```python
from build123d import *

# Parameters (mm, degrees)
SKETCH1_W           = 50.8
SKETCH1_H           = 25.4
BOSS_EXTRUDE2_DEPTH = 25.4
SKETCH3_R           = 5.08
BOSS_EXTRUDE3_DEPTH = 12.7
BOSS_EXTRUDE4_START = 50.8
BOSS_EXTRUDE4_DEPTH = 12.7
CUT_EXTRUDE1_START  = 58.42
CUT_EXTRUDE1_DEPTH  = 2.54
FILLET8_R           = 2.54


with BuildPart() as part:
    # Sketch1 → Boss-Extrude2 (new body)
    with BuildSketch(Plane(origin=(0, 0, 0), x_dir=(1, 0, 0), z_dir=(0, 1, 0))):
        with Locations((25.4, 12.7)):
            Rectangle(SKETCH1_W, SKETCH1_H)
    extrude(amount=BOSS_EXTRUDE2_DEPTH)

    # Sketch3 → Boss-Extrude3 (add)
    with BuildSketch(Plane.XY):
        with Locations(Location((12.7, 12.7, 0), (0, 0, 180))):
            Circle(SKETCH3_R)
        with Locations(Location((38.1, 12.7, 0), (0, 0, 180))):
            Circle(SKETCH3_R)
    extrude(amount=BOSS_EXTRUDE3_DEPTH)

    # Sketch4 → Boss-Extrude4 (add)
    with BuildSketch(Plane(origin=(0, 0, 0), x_dir=(0, 0, -1), z_dir=(1, 0, 0)).offset(BOSS_EXTRUDE4_START)):
        with BuildLine():
            Line((-6.35, 12.7), (6.35, 12.7))
            ThreePointArc((6.35, 12.7), (0, 6.35), (-6.35, 12.7))
        make_face()
    extrude(amount=BOSS_EXTRUDE4_DEPTH)

    # Sketch24 → Cut-Extrude1 (cut)
    with BuildSketch(Plane(origin=(0, 0, 0), x_dir=(0, 0, -1), z_dir=(1, 0, 0)).offset(CUT_EXTRUDE1_START)):
        with BuildLine():
            Line((-6.35, 12.7), (6.35, 12.7))
            ThreePointArc((6.35, 12.7), (0, 6.35), (-6.35, 12.7))
        make_face()
        with BuildLine():
            Line((-4.824854626, 11.43), (5.012523073, 11.43))
            ThreePointArc((5.012523073, 11.43), (0.093834223, 7.62), (-4.824854626, 11.43))
        make_face(mode=Mode.SUBTRACT)
    extrude(amount=CUT_EXTRUDE1_DEPTH, mode=Mode.SUBTRACT)

    # Fillet8
    fillet8_edges = [part.edges().sort_by_distance(p)[0] for p in [
        (50.8, 8.209871939, -4.490128061),
    ]]
    fillet(fillet8_edges, radius=FILLET8_R)


solid = part.part
```
CAD build for the part. Positions are in the model's coordinates, mm. A direction names the side the tool comes from. Round coordinates to 2 decimals unless told otherwise and drop trailing zeros. Order: outer loops, then holes, each group sorted by start corner. A loop starts at its lowest first (then second) coordinate and runs counter-clockwise, first axis right, second up. Notation, with made-up numbers: (34.25, 48.25) -> (68.25, 48.25) arc R12 ccw to (68.25, 60.25) -> close; hole circle Ø6 at (9, 3.5). An arc over 180 degrees is marked (long way). One line per question, with ' | ' between items.
Q1. Slice it at B-B (z = -20.5). Write the cut outline in (x, y).
Completed:
outline: (0, 0) -> (50.8, 0) -> (50.8, 25.4) -> (0, 25.4) -> close
Q2. Slice it at D-D (x = 13.5). Write the cut outline in (y, z), then the cut area to 3 significant figures.
Completed:
outline: (0, -25.4) -> (25.4, -25.4) -> (25.4, 0) -> (17.72, 0) -> (17.72, 12.7) -> (7.68, 12.7) -> (7.68, 0) -> (0, 0) -> close | area: 773 mm^2
Q3. Slice it at A-A (x = 38.1). Write the cut outline in (y, z), then the cut area to 3 significant figures.
Completed:
outline: (0, -25.4) -> (25.4, -25.4) -> (25.4, 0) -> (17.78, 0) -> (17.78, 12.7) -> (7.62, 12.7) -> (7.62, 0) -> (0, 0) -> close | area: 774 mm^2
Q4. Drop flat-ended pins along their axis: pin 1 (4 mm diameter, centred on x = 55, z = -1.5, fed in from +Y); pin 2 (3 mm diameter, centred on y = 10.5, z = 2, fed in from -X); pin 3 (5 mm diameter, centred on x = 32.5, z = 8, fed in from +Y). Give the stop position or say it passes through.
Completed:
pin 1: stops at y = 12.7 | pin 2: stops at x = 7.67 | pin 3: stops at y = 16.72
Q5. Probe probe 1 along X at (y, z) = (20, -17); probe 2 along Z at (x, y) = (7, 19); probe 3 along Y at (x, z) = (51.5, -2.5). List the from-to ranges inside material, lowest first.
Completed:
probe 1: x = 0 to 50.8 | probe 2: z = -25.4 to 0 | probe 3: y = 6.01 to 12.7
Q6. Which spindle directions (+Z, -Z, +X, -X, +Y, -Y) get a long thin tool onto all of the face, cutting with end or side? Do faces 5 (the cylindrical face through (62.21, 6.35, -0.14)), 6 (the flat face through (50.8, 10, 2)), 7 (the flat face through (62, 12.7, 0)), 8 (the cylindrical face through (13.8, 17.66, 6.26)). Say none if no direction does.
Completed:
face 5: +X, -Y | face 6: +Z, +Y, -Y | face 7: +Z, -Z, +X, +Y | face 8: +Z
Q7. Slice it at C-C (y = 21.25). Write the cut outline in (x, z).
Completed:
outline: (0, -25.4) -> (50.8, -25.4) -> (50.8, 0) -> (0, 0) -> close
Q8. Two-plate mould, pull along X, no slides. Class faces 1 (the flat face through (60, 11.43, 0)), 2 (the flat face through (58.42, 12, 0)), 3 (the flat face through (13, 13, 12.7)), 4 (the flat face through (63.5, 10, 0)): released by +X, released by -X, zero draft, split by the parting line, or undercut.
Completed:
face 1: undercut | face 2: undercut | face 3: zero draft | face 4: released by +X
